Design review of the part shown in the three views and the two pictorial views. Dimensions are in mm from the part's minimum x, y and z. A direction names the side the tool comes from. Give positions to 0.01 mm unless a question says otherwise; leave off trailing zeros. Order: outer loops, then holes, each group sorted by start corner. A loop starts at its lowest first (then second) coordinate and runs counter-clockwise, first axis right, second up.
Item 1: Consider section D-D (y = 20). Give the boundary of the cut face in (x, z) (1 decimal).
Item 2: The part is to be moulded in two halves that separate along X. For the marked faces 1, 2 and 3, say which applies: released by +X, released by -X, zero draft, split by the parting line, or undercut.
Item 3: Consider section A-A (y = 50). Give the boundary of the cut face in (x, z) (1 decimal), plus the area to 3 significant figures.
Item 4: Consider section C-C (z = 37.5). Give the boundary of the cut face in (x, y) (1 decimal).
Item 5: For P1, Ø6.5, axis at x = 104.5, y = 13.5, coming from the -Z side; P2, Ø4, axis at y = 52, z = 9, coming from the +X side, all flat-tipped, find the tip position at first contact; note any pin that passes through.
Item 6: Consider section B-B (x = 110.5). Give the boundary of the cut face in (y, z), plus the area to 4 significant figures.
Item 7: For probe 1 along Y at (x, z) = (92, 39.5) (1 decimal); probe 2 along X at (y, z) = (50, 17) (1 decimal); probe 3 along X at (y, z) = (50, 25) (1 decimal), list the stretches that pass through material, from the lowest coordinate up.
Item 8: Machinability: for the marked faces 4, 5 and 6, which of the approach directions +Z, -Z, +X, -X, +Y, -Y give a long, thin tool a straight path to every point of the face, cutting with its end or side? Answer none if there is none.
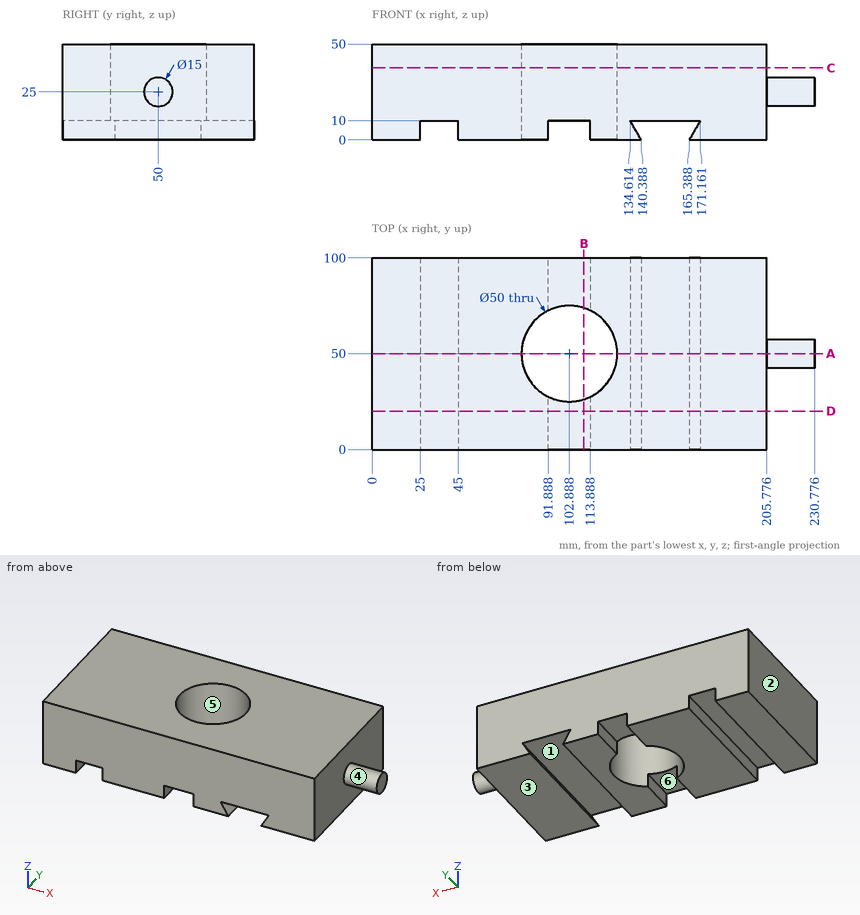
Resolved:
1. outline: (0, 0) - (25, 0) - (25, 10) - (45, 10) - (45, 0) - (91.9, 0) - (91.9, 10) - (113.9, 10) - (113.9, 0) - (140.4, 0) - (134.6, 10) - (171.2, 10) - (165.4, 0) - (205.8, 0) - (205.8, 50) - (0, 50) - close
2. face 1: undercut
2. face 2: released by -X
2. face 3: zero draft
3. outline: (0, 0) - (25, 0) - (25, 10) - (45, 10) - (45, 0) - (77.9, 0) - (77.9, 50) - (0, 50) - close; (127.9, 0) - (140.4, 0) - (134.6, 10) - (171.2, 10) - (165.4, 0) - (205.8, 0) - (205.8, 17.5) - (230.8, 17.5) - (230.8, 32.5) - (205.8, 32.5) - (205.8, 50) - (127.9, 50) - close
3. area: 7,660 mm2
4. outline: (0, 0) - (205.8, 0) - (205.8, 100) - (0, 100) - close; hole circle Ø50 at (102.9, 50)
5. P1: stops at z = 10
5. P2: stops at x = 205.78
6. outline: (0, 10) - (26.19, 10) - (26.19, 50) - (0, 50) - close; (73.81, 10) - (100, 10) - (100, 50) - (73.81, 50) - close
6. area: 2,095 mm2
7. probe 1: y = 0 to 27.5, 72.5 to 100
7. probe 2: x = 0 to 77.9, 127.9 to 205.8
7. probe 3: x = 0 to 77.9, 127.9 to 230.8
8. face 4: +X
8. face 5: +Z, -Z
8. face 6: -Z, +Y, -Y
